The figure shows three views and two pictorial views of one solid part (mm, origin at its lowest corner). Answer the questions. A direction names the side the tool comes from. Give positions to 0.01 mm unless a question says otherwise; leave off trailing zeros. Loops run counter-clockwise (first coordinate to the right, second up) from the corner with the lowest first, then second, coordinate; pieces in that order, holes last. Notation, with made-up numbers: (66, -30.75) - (95, -30.75) arc R25 cw to (95, -11.75) - close; hole circle Ø8 at (-32, 5). An arc over 180 degrees is marked (long way). Write item = value, one per line.
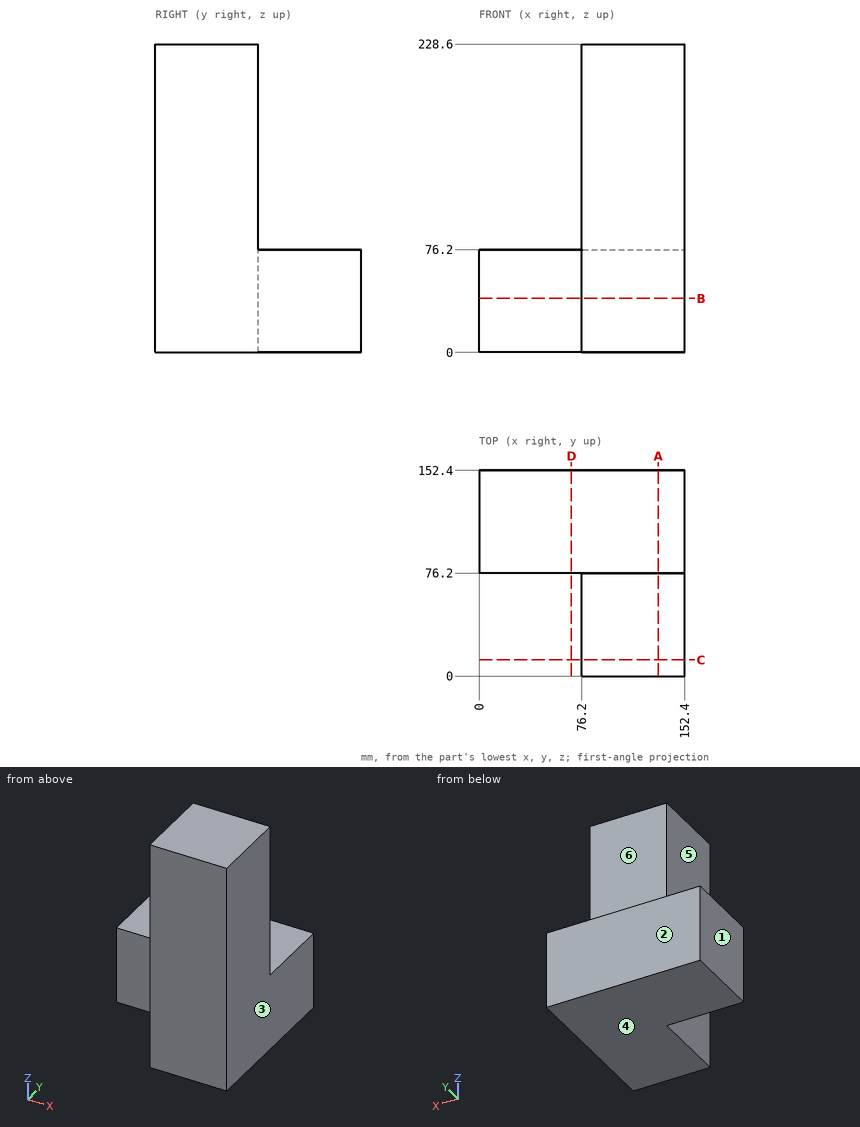
1) Each of these flat-tipped pins is pushed along its axis until it touches: P1, Ø5, axis at x = 134, y = 80.5, coming from the +Z side; P2, Ø2, axis at y = 17.5, z = 23.5, coming from the -X side; P3, Ø23, axis at x = 33, z = 36.5, coming from the -Y side. Where does it stop, or does it pass through?
Output:
P1 = 76.2
P2 = 76.2
P3 = 76.2
2) A cutting plane is placed at D-D on x = 68.5. Determine the outline of the cut face in (y, z).
Output:
outline = (76.2, 0) - (152.4, 0) - (152.4, 76.2) - (76.2, 76.2) - close
3) A cutting plane is placed at B-B on z = 40. Determine the outline of the cut face in (x, y), then the cut area to 3 significant figures.
Output:
outline = (0, 76.2) - (76.2, 76.2) - (76.2, 0) - (152.4, 0) - (152.4, 152.4) - (0, 152.4) - close
area = 17,400 mm²
4) Find the intervals of material crossed by probe 1 along Z at (x, y) = (135.5, 140); probe 2 along Y at (x, z) = (62.5, 51), in increasing order.
Output:
probe_1 = 0 to 76.2
probe_2 = 76.2 to 152.4
5) The mould has two halves that part along X. Classify the marked faces 1, 2 and 3: pulls with the +X half, pulls with the -X half, needs draft (parallel to the pull), parting line crosses it, or undercut.
Output:
face_1 = pulls with the -X half
face_2 = needs draft
face_3 = pulls with the +X half
6) A cutting plane is placed at C-C on y = 12. Determine the outline of the cut face in (x, z), then the cut area to 3 significant figures.
Output:
outline = (76.2, 0) - (152.4, 0) - (152.4, 228.6) - (76.2, 228.6) - close
area = 17,400 mm²
7) A tool of negligible diameter and unlimited length cuts with its end or side. For the marked faces 4, 5 and 6, from which of +Z, -Z, +X, -X, +Y, -Y can it reach the whole face along a straight path? Write none if from no direction.
Output:
face_4 = -Z, +X, -X, +Y, -Y
face_5 = +Z, -Z, -X, -Y
face_6 = +Z, +X, -X, +Y
8) A cutting plane is placed at A-A on x = 133. Determine the outline of the cut face in (y, z).
Output:
outline = (0, 0) - (152.4, 0) - (152.4, 76.2) - (76.2, 76.2) - (76.2, 228.6) - (0, 228.6) - close
